The drawing under review shows one solid part. Ordinate dimensions are in mm from its lowest x, y, z. A direction names the side the tool comes from. Round coordinates to 2 decimals unless told otherwise and drop trailing zeros. Order: outer loops, then holes, each group sorted by start corner. A loop starts at its lowest first (then second) coordinate and runs counter-clockwise, first axis right, second up. Notation, with made-up numbers: M 88.5,-21 L 118.5,-21 A12 cw 118.5,-16 Z; hole C 77,44.5 d9. An arc over 180 degrees is marked long. Answer as a JSON object with one key per item and string values. Group by question number.
1) Consider section A-A, the plane x = 56. Write out the cut boundary in (y, z), then the cut area to 3 significant figures.
2) Insertion check: pin 1 Ø2 at (y, z) = (11.5, 7.5) entering from +X; pin 2 Ø19.5 at (x, z) = (25, 54.13) entering from +Y; pin 3 Ø2 at (x, y) = (29, 31.5) entering from -Z; pin 4 Ø6 at (x, y) = (63, 16) entering from -Z. Each pin has a flat end and moves straight along its axis. Give the tip position at first contact, or say it passes through.
3) Consider section B-B, the plane y = 23.5. Write out the cut boundary in (x, z).
4) To check wall thickness, follow line 1 (Z direction, x = 50, y = 31.5); line 2 (X direction, y = 10, z = 59.5); line 3 (X direction, y = 17.5, z = 48.5). State the ranges of each line that lie inside material, in increasing order.
5) Consider section D-D, the plane z = 39. Write out the cut boundary in (x, y), then the cut area to 3 significant figures.
6) Consider section C-C, the plane x = 20. Write out the cut boundary in (y, z).
7) For the marked faces 5 and 6, list the 3-axis set-ups (+Z, -Z, +X, -X, +Y, -Y) from which the entire face can be reached by the end or side of a thin tool; tool diameter is ignored.
8) The part is to be moulded in two halves that separate along X. For the marked faces 1, 2, 3 and 4, say which applies: +X half, -X half, draft (parallel to the pull), parting line (faces both ways), or undercut.
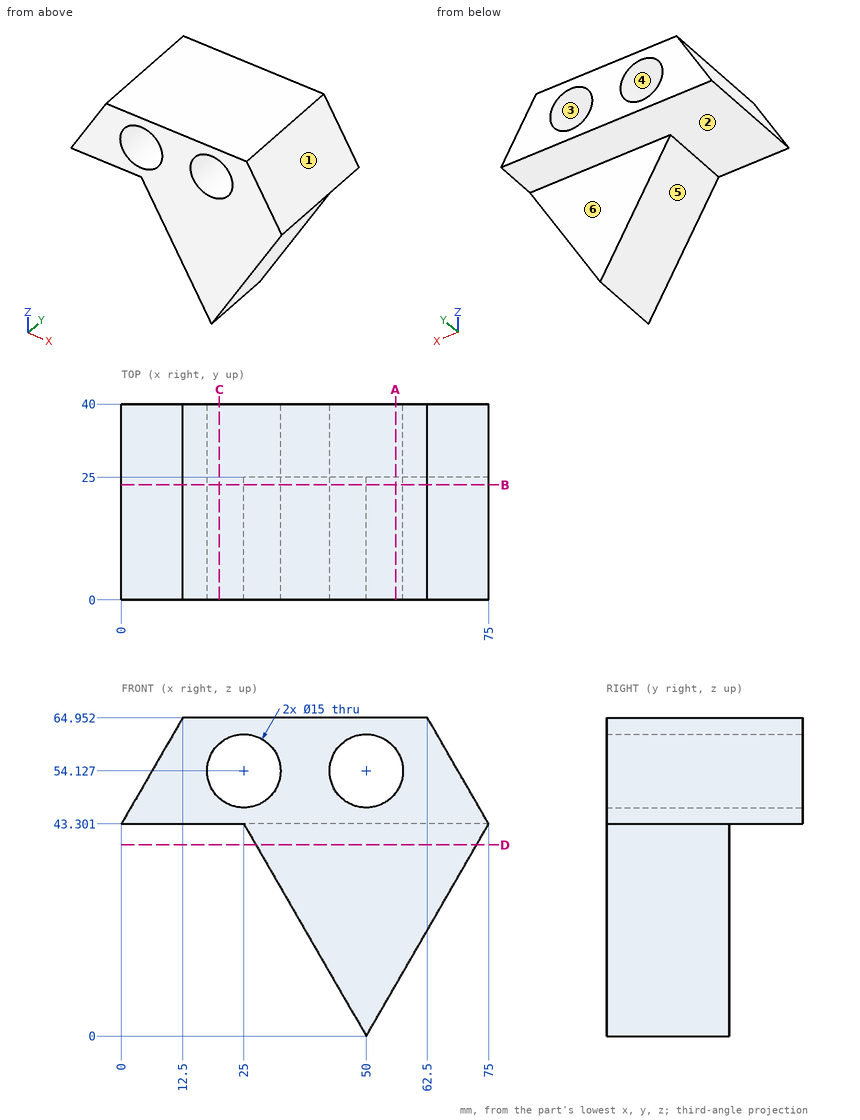
Results list:
{
 "1": {"outline": "M 0,10.39 L 25,10.39 L 25,43.3 L 40,43.3 L 40,49.63 L 0,49.63 Z; M 0,58.63 L 40,58.63 L 40,64.95 L 0,64.95 Z", "area": "1,330 mm^2"},
 "2": {"pin 1": "x = 54.91", "pin 2": "y = 40", "pin 3": "z = 43.3", "pin 4": "z = 17.32"},
 "3": {"outline": "M 0,43.3 L 25,43.3 L 50,0 L 75,43.3 L 62.5,64.95 L 12.5,64.95 Z; hole C 25,54.13 d15; hole C 50,54.13 d15"},
 "4": {"line 1": "43.3 to 46.63, 61.63 to 64.95", "line 2": "9.35 to 19.77, 30.23 to 44.77, 55.23 to 65.65", "line 3": "3 to 20.04, 29.96 to 45.04, 54.96 to 72"},
 "5": {"outline": "M 27.48,0 L 72.52,0 L 72.52,25 L 27.48,25 Z", "area": "1,130 mm^2"},
 "6": {"outline": "M 0,43.3 L 40,43.3 L 40,48.54 L 0,48.54 Z; M 0,59.72 L 40,59.72 L 40,64.95 L 0,64.95 Z"},
 "7": {"face 5": "-Z, -X, +Y, -Y", "face 6": "-Z, +X, -X, +Y"},
 "8": {"face 1": "+X half", "face 2": "draft", "face 3": "undercut", "face 4": "undercut"}
}
